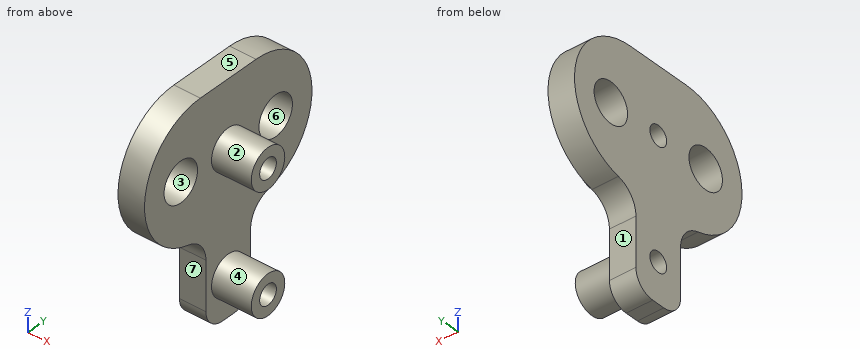
```python
from build123d import *

# Parameters (mm, degrees)
BOSS_EXTRUDE1_DEPTH      = 4
SKETCH2_W                = 6
SKETCH2_H                = 3
SKETCH3_W                = 6
SKETCH3_H                = 3
F_3_0_3_DIAMETER_HOLE1_D = 3
F_6_0_6_DIAMETER_HOLE1_D = 6
FILLET1_R                = 3
FILLET2_R                = 4


with BuildPart() as part:
    # Sketch1 → Boss-Extrude1 (new body)
    with BuildSketch(Plane(origin=(24, 0, 0), x_dir=(0, 0, -1), z_dir=(1, 0, 0))):
        with BuildLine():
            Line((-96.043137062, 96.972273827), (-110.093262691, 96.972273827))
            ThreePointArc((-110.093262691, 96.972273827), (-119.542509311, 107.959734558), (-130.043137062, 97.972273827))
            Line((-130.043137062, 97.972273827), (-130.043137062, 87.972273827))
            ThreePointArc((-130.043137062, 87.972273827), (-119.542509311, 77.984813095), (-110.093262691, 88.972273827))
            Line((-110.093262691, 88.972273827), (-96.043137062, 88.972273827))
            Line((-96.043137062, 88.972273827), (-96.043137062, 96.972273827))
        make_face()
    extrude(amount=-BOSS_EXTRUDE1_DEPTH)

    # Sketch2 → Revolve1 (revolve)
    with BuildSketch(Plane.XY.offset(102.043137062), mode=Mode.PRIVATE) as revolve1_sk:
        with Locations((27, 94.472273827)):
            Rectangle(SKETCH2_W, SKETCH2_H)
    revolve(revolve1_sk.sketch.rotate(Axis((24, 92.972273827, 102.043137062), (1, 0, 0)), 270), axis=Axis((24, 92.972273827, 102.043137062), (1, 0, 0)))

    # Sketch3 → Revolve2 (revolve)
    with BuildSketch(Plane.XY.offset(120.043137062), mode=Mode.PRIVATE) as revolve2_sk:
        with Locations((27, 94.472273827)):
            Rectangle(SKETCH3_W, SKETCH3_H)
    revolve(revolve2_sk.sketch.rotate(Axis((24, 92.972273827, 120.043137062), (1, 0, 0)), 270), axis=Axis((24, 92.972273827, 120.043137062), (1, 0, 0)))

    # Ø3.0 (3) Diameter Hole1 (through all)
    with Locations(Plane(origin=(30, 0, 0), x_dir=(0, 0, -1), z_dir=(1, 0, 0))):
        with Locations((-120.043137062, 92.972273827), (-102.043137062, 92.972273827)):
            Hole(F_3_0_3_DIAMETER_HOLE1_D / 2)

    # Ø6.0 (6) Diameter Hole1 (through all)
    with Locations(Plane(origin=(24, 0, 0), x_dir=(0, 0, -1), z_dir=(1, 0, 0))):
        with Locations((-120.043137062, 101.472273827), (-120.043137062, 84.472273827)):
            Hole(F_6_0_6_DIAMETER_HOLE1_D / 2)

    # Fillet1
    fillet1_edges = [part.edges().sort_by_distance(p)[0] for p in [
        (22, 88.972273827, 96.043137062),
        (22, 96.972273827, 96.043137062),
    ]]
    fillet(fillet1_edges, radius=FILLET1_R)

    # Fillet2
    fillet2_edges = [part.edges().sort_by_distance(p)[0] for p in [
        (22, 88.972273827, 110.093262691),
        (22, 96.972273827, 110.093262691),
    ]]
    fillet(fillet2_edges, radius=FILLET2_R)


solid = part.part
```
Input: part model. Units: mm. Frame: model coordinates. Face numbers are marked on the shaded views. A direction names the side the tool comes from. Round coordinates to 2 decimals unless told otherwise and drop trailing zeros. Order: outer loops, then holes, each group sorted by start corner. A loop starts at its lowest first (then second) coordinate and runs counter-clockwise, first axis right, second up. Notation, with made-up numbers: (-13.75, 30.25) - (-1.75, 30.25) arc R4 cw to (-1.75, 37.25) - close; hole circle Ø3 at (84.5, -15). An arc over 180 degrees is marked (long way). Answer in a Markdown table with one row per item.
Item 1: Section query A-A (z = 101). Return the cut outline in (x, y), then the cut area to 3 significant figures.
Model answer:
| item | result |
|---|---|
| outline | (20, 88.97) - (24, 88.97) - (24, 90.16) - (30, 90.16) - (30, 91.89) - (20, 91.89) - close; (20, 94.05) - (30, 94.05) - (30, 95.79) - (24, 95.79) - (24, 96.97) - (20, 96.97) - close |
| area | 44.2 mm² |
Item 2: Section query B-B (x = 21). Return the cut outline in (y, z).
Model answer:
| item | result |
|---|---|
| outline | (85.83, 110.28) arc R4 cw to (88.97, 106.37) - (88.97, 99.04) arc R3 ccw to (91.97, 96.04) - (93.97, 96.04) arc R3 ccw to (96.97, 99.04) - (96.97, 106.37) arc R4 cw to (100.12, 110.28) arc R10 ccw to (97.97, 130.04) - (87.97, 130.04) arc R10 ccw to start; hole circle Ø6 at (84.47, 120.04); hole circle Ø3 at (92.97, 102.04); hole circle Ø3 at (92.97, 120.04); hole circle Ø6 at (101.47, 120.04) |
Item 3: Line query: line 1 (X direction, y = 105.5, z = 118.5); line 2 (Z direction, x = 29.5, y = 95); line 3 (Z direction, x = 20.75, y = 99.5). Output: solid intervals per line, ascending.
Model answer:
| item | result |
|---|---|
| line 1 | x = 20 to 24 |
| line 2 | z = 99.83 to 104.25, 117.83 to 122.25 |
| line 3 | z = 110.09 to 117.78, 122.3 to 129.93 |
Item 4: Mould query, pull axis Z, two halves, no side actions, for the marked faces 4, 5, 6 and 7. Classes: released by +Z, released by -Z, zero draft, split by the parting line, or undercut.
Model answer:
| item | result |
|---|---|
| face 4 | undercut |
| face 5 | released by +Z |
| face 6 | undercut |
| face 7 | zero draft |
Item 5: Section query C-C (y = 104). Return the cut outline in (x, z).
Model answer:
| item | result |
|---|---|
| outline | (20, 112.06) - (24, 112.06) - (24, 118.43) - (20, 118.43) - close; (20, 121.66) - (24, 121.66) - (24, 128.02) - (20, 128.02) - close |
Item 6: Section query D-D (y = 91). Return the cut outline in (x, z), then the cut area to 3 significant figures.
Model answer:
| item | result |
|---|---|
| outline | (20, 96.21) - (24, 96.21) - (24, 99.78) - (30, 99.78) - (30, 104.3) - (24, 104.3) - (24, 117.78) - (30, 117.78) - (30, 122.3) - (24, 122.3) - (24, 130.04) - (20, 130.04) - close |
| area | 190 mm² |
Item 7: Pin query (flat end, axial travel): pin 1 (3 mm diameter, centred on x = 21.5, z = 124.5, fed in from -Y); pin 2 (5 mm diameter, centred on x = 24.5, y = 91, fed in from -Z); pin 3 (5 mm diameter, centred on y = 84.47, z = 120.04, fed in from -X); pin 4 (9 mm diameter, centred on y = 94.5, z = 110, fed in from +X). Return the tip coordinate at first contact, or that it passes through.
Model answer:
| item | result |
|---|---|
| pin 1 | stops at y = 78.42 |
| pin 2 | stops at z = 96.04 |
| pin 3 | passes through |
| pin 4 | stops at x = 24 |
Item 8: Reachability of the marked faces 1, 2 and 3 from +Z, -Z, +X, -X, +Y, -Y: full face, straight path, thin tool, end or side. Return the list, or none.
Model answer:
| item | result |
|---|---|
| face 1 | -Z, +X, -X, +Y |
| face 2 | +X |
| face 3 | +X, -X |
